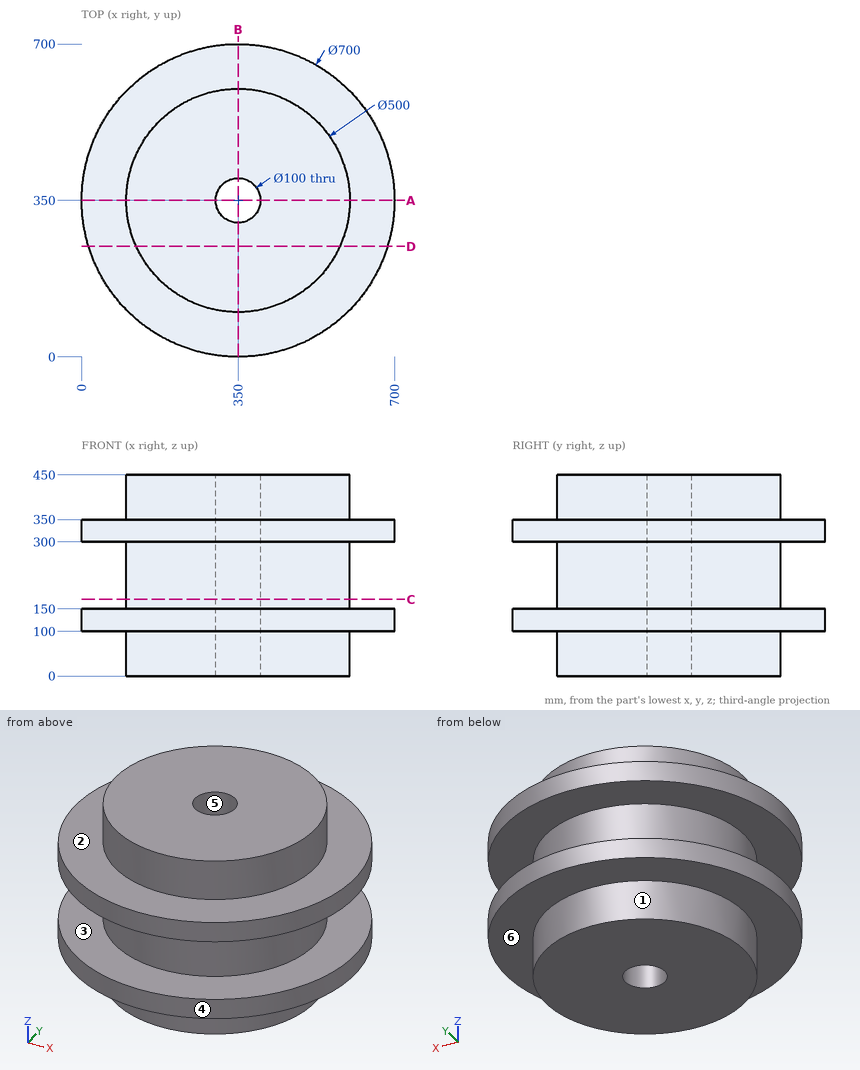
Part print with two shaded views. Sizes in mm from the minimum x, y, z corner. A direction names the side the tool comes from. Round coordinates to 2 decimals unless told otherwise and drop trailing zeros. Order: outer loops, then holes, each group sorted by start corner. A loop starts at its lowest first (then second) coordinate and runs counter-clockwise, first axis right, second up.
(1) Band-saw the part on C-C (z = 171.5). List the corners of the cut face in (x, y), then the cut area to 3 significant figures.
(2) Pin check, flat tips, straight feed: pin 1 (3 mm diameter, centred on x = 295, z = 89.5, fed in from -Y); pin 2 (10 mm diameter, centred on y = 404.5, z = 305.5, fed in from +X); pin 3 (2 mm diameter, centred on y = 451.5, z = 76.5, fed in from -X). Stop position of each tip, or through.
(3) Pull direction X, two halves, no side cores. Call the marked faces 4, 5 and 6: released by +X, released by -X, zero draft, split by the parting line, or undercut.
(4) 3-axis set-ups, long thin cutter, end or side, ignore diameter. For the marked faces 1, 2 and 3: which of +Z, -Z, +X, -X, +Y, -Y reach the whole face in a straight line?
(5) Drill centre lines: line 1 (Z direction, x = 84, y = 152); line 2 (Y direction, x = 350, z = 318); line 3 (Y direction, x = 350, z = 299). Where is each one in solid material? Low to high.
(6) Band-saw the part on D-D (y = 247). List the corners of the cut face in (x, z), then the cut area to 3 significant figures.
(7) Band-saw the part on A-A (y = 350). List the corners of the cut face in (x, z).
Verdict:
1. outline: circle Ø500 at (350, 350); hole circle Ø100 at (350, 350)
1. area: 188,000 mm2
2. pin 1: stops at y = 105.79
2. pin 2: stops at x = 696.48
2. pin 3: stops at x = 121.09
3. face 4: split by the parting line
3. face 5: undercut
3. face 6: zero draft
4. face 1: -Z
4. face 2: +Z
4. face 3: none
5. line 1: z = 100 to 150, 300 to 350
5. line 2: y = 0 to 300, 400 to 700
5. line 3: y = 100 to 300, 400 to 600
6. outline: (15.5, 100) - (122.2, 100) - (122.2, 0) - (577.8, 0) - (577.8, 100) - (684.5, 100) - (684.5, 150) - (577.8, 150) - (577.8, 300) - (684.5, 300) - (684.5, 350) - (577.8, 350) - (577.8, 450) - (122.2, 450) - (122.2, 350) - (15.5, 350) - (15.5, 300) - (122.2, 300) - (122.2, 150) - (15.5, 150) - close
6. area: 226,000 mm2
7. outline: (0, 100) - (100, 100) - (100, 0) - (300, 0) - (300, 450) - (100, 450) - (100, 350) - (0, 350) - (0, 300) - (100, 300) - (100, 150) - (0, 150) - close; (400, 0) - (600, 0) - (600, 100) - (700, 100) - (700, 150) - (600, 150) - (600, 300) - (700, 300) - (700, 350) - (600, 350) - (600, 450) - (400, 450) - close
